```python
from build123d import *

# Parameters (mm, degrees)
F1_DEPTH      = 9
F2_R          = 5
F3_DEPTH      = 25
F4_W          = 103.9993347282
F4_H          = 56.6140824735
F5_DEPTH      = 25
F6_W          = 113.1558813547
F6_H          = 45.2373955332
F7_DEPTH      = 25
F8_R          = 5
F9_SIZE       = 5
F10_R         = 10
F11_T1_DEPTH  = 37.8584149398
F11_T3_DEPTH  = 109.8584149398
F11_T5_DEPTH  = 56.6140824735
F11_T7_DEPTH  = 104.1027474062
F11_T9_DEPTH  = 322.7168298797
F11_T11_DEPTH = 45.7168298797
F11_T13_DEPTH = 112.8584149398
F11_T15_DEPTH = 45.2373955332
F11_T17_DEPTH = 107.6210194067
F11_T19_DEPTH = 197
F11_T22_ANGLE = 90
F11_T24_ANGLE = 90
F11_T29_DEPTH = 122.7168298797
F11_T33_DEPTH = 69.4724974133
F11_T40_DEPTH = 69.4724974133
F11_T44_DEPTH = 122.7168298797
F11_T51_DEPTH = 58.095810473
F11_T55_DEPTH = 125.7168298797
F11_T62_DEPTH = 125.7168298797
F11_T66_DEPTH = 58.095810473


# Not quite as in the source:
# - a fillet or chamfer that OpenCascade refuses, or shapes differently, is made with other operations: its cross-section is extruded or revolved along the edge and cut away or added


with BuildPart() as f1:
    # F0 (on Front) → F1 (new body)
    with BuildSketch(Plane.XZ):
        with BuildLine():
            Line((100.0664040952, 56.5429037459), (-96.9335959048, 56.5429037459))
            ThreePointArc((-96.9335959048, 56.5429037459), (-132.2889349642, 41.8982428052), (-146.9335959048, 6.5429037459))
            Line((-146.9335959048, 6.5429037459), (-146.9335959048, -153.4570962541))
            Line((-146.9335959048, -153.4570962541), (150.0664040952, -153.4570962541))
            Line((150.0664040952, -153.4570962541), (150.0664040952, 6.5429037459))
            ThreePointArc((150.0664040952, 6.5429037459), (135.4217431545, 41.8982428052), (100.0664040952, 56.5429037459))
        make_face()
    extrude(amount=F1_DEPTH)

    # F2 (on face) → F3 (join)
    with BuildSketch(Plane.XZ.offset(9)):
        with Locations((-46.9335959048, -43.4570962541)):
            Circle(F2_R)
        with Locations((-96.9335959048, -43.4570962541)):
            Circle(F2_R)
    extrude(amount=F3_DEPTH)

    # F4 (on face) → F5 (cut)
    with BuildSketch(Plane.XZ.offset(9)):
        with Locations((105.0660714593, -46.7641374908)):
            Rectangle(F4_W, F4_H)
    extrude(amount=-F5_DEPTH, mode=Mode.SUBTRACT)

    # F6 (on face) → F7 (cut)
    with BuildSketch(Plane.XZ.offset(9)):
        with Locations((-103.5115365822, -110.8383984875)):
            Rectangle(F6_W, F6_H)
    extrude(amount=-F7_DEPTH, mode=Mode.SUBTRACT)

    # F8
    f8_edges = [f1.edges().sort_by_distance(p)[0] for p in [
        (150.066404, -9, -5.957096),
        (101.566404, -9, -18.457096),
        (53.066404, -9, -46.764137),
        (101.566404, -9, -75.071179),
        (150.066404, -9, -114.264137),
        (1.566404, -9, -153.457096),
        (-146.933596, -9, -143.457096),
        (-96.933596, -9, -133.457096),
        (-46.933596, -9, -110.838398),
        (-96.933596, -9, -88.219701),
        (-146.933596, -9, -40.838398),
        (-132.288935, -9, 41.898243),
        (1.566404, -9, 56.542904),
        (135.421743, -9, 41.898243),
        (-101.933596, -9, -43.457096),
        (-51.933596, -9, -43.457096),
    ]]
    fillet(f8_edges, radius=F8_R)

    # F9
    f9_edges = [f1.edges().sort_by_distance(p)[0] for p in [
        (-101.933596, -34, -43.457096),
        (-51.933596, -34, -43.457096),
    ]]
    chamfer(f9_edges, length=F9_SIZE)

    # F10
    f10_edges = [f1.edges().sort_by_distance(p)[0] for p in [
        (-94.433596, -31.5, -43.457096),
        (-101.933596, -29, -43.457096),
        (-44.433596, -31.5, -43.457096),
        (-51.933596, -29, -43.457096),
    ]]
    fillet(f10_edges, radius=F10_R)

    # F11: chamfer of 5 on 14 edges, made by hand

    # F11_s2 → F11_t1 (cut)
    with BuildSketch(Plane.XY.offset(-31.3155111939)):
        Polygon((150.0664040952, -5), (145.0664040952, 0), (150.0664040952, 0), align=None)
    extrude(amount=F11_T1_DEPTH, mode=Mode.SUBTRACT)

    # F11_s4 → F11_t3 (cut)
    with BuildSketch(Plane.YZ.offset(53.0664040952)):
        Polygon((-5, -18.4570962541), (0, -13.4570962541), (0, -18.4570962541), align=None)
        Polygon((-5, -75.0711787276), (0, -80.0711787276), (0, -75.0711787276), align=None)
    extrude(amount=F11_T3_DEPTH, mode=Mode.SUBTRACT)

    # F11_s6 → F11_t5 (cut)
    with BuildSketch(Plane.XY.offset(-75.0711787276)):
        Polygon((53.0664040952, -5), (48.0664040952, 0), (53.0664040952, 0), align=None)
    extrude(amount=F11_T5_DEPTH, mode=Mode.SUBTRACT)

    # F11_s8 → F11_t7 (cut)
    with BuildSketch(Plane.XY.offset(-166.3155111939)):
        Polygon((150.0664040952, -5), (145.0664040952, 0), (150.0664040952, 0), align=None)
    extrude(amount=F11_T7_DEPTH, mode=Mode.SUBTRACT)

    # F11_s10 → F11_t9 (cut)
    with BuildSketch(Plane.YZ.offset(-159.7920108447)):
        Polygon((-5, -153.4570962541), (0, -148.4570962541), (0, -153.4570962541), align=None)
    extrude(amount=F11_T9_DEPTH, mode=Mode.SUBTRACT)

    # F11_s12 → F11_t11 (cut)
    with BuildSketch(Plane.XY.offset(-166.3155111939)):
        Polygon((-146.9335959048, -5), (-141.9335959048, 0), (-146.9335959048, 0), align=None)
    extrude(amount=F11_T11_DEPTH, mode=Mode.SUBTRACT)

    # F11_s14 → F11_t13 (cut)
    with BuildSketch(Plane.YZ.offset(-159.7920108447)):
        Polygon((-5, -133.4570962541), (0, -138.4570962541), (0, -133.4570962541), align=None)
        Polygon((-5, -88.2197007209), (0, -83.2197007209), (0, -88.2197007209), align=None)
    extrude(amount=F11_T13_DEPTH, mode=Mode.SUBTRACT)

    # F11_s16 → F11_t15 (cut)
    with BuildSketch(Plane.XY.offset(-133.4570962541)):
        Polygon((-46.9335959048, -5), (-41.9335959048, 0), (-46.9335959048, 0), align=None)
    extrude(amount=F11_T15_DEPTH, mode=Mode.SUBTRACT)

    # F11_s18 → F11_t17 (cut)
    with BuildSketch(Plane.XY.offset(-101.0781156608)):
        Polygon((-146.9335959048, -5), (-141.9335959048, 0), (-146.9335959048, 0), align=None)
    extrude(amount=F11_T17_DEPTH, mode=Mode.SUBTRACT)

    # F11_s20 → F11_t19 (cut)
    with BuildSketch(Plane.YZ.offset(-96.9335959048)):
        Polygon((-5, 56.5429037459), (0, 51.5429037459), (0, 56.5429037459), align=None)
    extrude(amount=F11_T19_DEPTH, mode=Mode.SUBTRACT)

    # F11_s21 → F11_t22 (revolve, cut)
    with BuildSketch(Plane.YZ.offset(-96.9335959048)):
        Polygon((-5, 56.5429037459), (0, 51.5429037459), (0, 56.5429037459), align=None)
    revolve(axis=Axis((-96.9335959048, 0, 6.5429037459), (0, -1, 0)), revolution_arc=F11_T22_ANGLE, mode=Mode.SUBTRACT)

    # F11_s23 → F11_t24 (revolve, cut)
    with BuildSketch(Plane.XY.offset(6.5429037459)):
        Polygon((150.0664040952, -5), (145.0664040952, 0), (150.0664040952, 0), align=None)
    revolve(axis=Axis((100.0664040952, 0, 6.5429037459), (0, -1, 0)), revolution_arc=F11_T24_ANGLE, mode=Mode.SUBTRACT)


with BuildPart() as f11_tool27:
    # F11_s28 → F11_t29 (new body)
    with BuildSketch(Plane.YZ.offset(162.924819035)):
        Polygon((-5, -18.4570962541), (0, -13.4570962541), (0, -18.4570962541), align=None)
    extrude(amount=-F11_T29_DEPTH)

    split(bisect_by=Plane.YZ.offset(53.0664040952), keep=Keep.BOTTOM)


with BuildPart() as f11_tool31:
    # F11_s32 → F11_t33 (new body)
    with BuildSketch(Plane.XY.offset(-5.5986813143)):
        Polygon((53.0664040952, -5), (48.0664040952, 0), (53.0664040952, 0), align=None)
    extrude(amount=-F11_T33_DEPTH)

    split(bisect_by=Plane.XY.offset(-18.4570962541), keep=Keep.TOP)


with BuildPart() as f11_tool27_1:
    add(f11_tool27.part)

    # F11_t35: intersect F11_tool31
    add(f11_tool31.part, mode=Mode.INTERSECT)


with BuildPart() as f1_1:
    add(f1.part)

    # F11_t25: cut F11_tool27
    add(f11_tool27_1.part, mode=Mode.SUBTRACT)


with BuildPart() as f11_tool38:
    # F11_s39 → F11_t40 (new body)
    with BuildSketch(Plane.XY.offset(-18.4570962541)):
        Polygon((53.0664040952, -5), (48.0664040952, 0), (53.0664040952, 0), align=None)
    extrude(amount=-F11_T40_DEPTH)

    split(bisect_by=Plane.XY.offset(-75.0711787276), keep=Keep.BOTTOM)


with BuildPart() as f11_tool42:
    # F11_s43 → F11_t44 (new body)
    with BuildSketch(Plane.YZ.offset(40.2079891553)):
        Polygon((-5, -75.0711787276), (0, -80.0711787276), (0, -75.0711787276), align=None)
    extrude(amount=F11_T44_DEPTH)

    split(bisect_by=Plane.YZ.offset(53.0664040952), keep=Keep.BOTTOM)


with BuildPart() as f11_tool38_1:
    add(f11_tool38.part)

    # F11_t46: intersect F11_tool42
    add(f11_tool42.part, mode=Mode.INTERSECT)


with BuildPart() as f1_2:
    add(f1_1.part)

    # F11_t36: cut F11_tool38
    add(f11_tool38_1.part, mode=Mode.SUBTRACT)


with BuildPart() as f11_tool49:
    # F11_s50 → F11_t51 (new body)
    with BuildSketch(Plane.XY.offset(-146.3155111939)):
        Polygon((-46.9335959048, -5), (-41.9335959048, 0), (-46.9335959048, 0), align=None)
    extrude(amount=F11_T51_DEPTH)

    split(bisect_by=Plane.XY.offset(-133.4570962541), keep=Keep.BOTTOM)


with BuildPart() as f11_tool53:
    # F11_s54 → F11_t55 (new body)
    with BuildSketch(Plane.YZ.offset(-159.7920108447)):
        Polygon((-5, -133.4570962541), (0, -138.4570962541), (0, -133.4570962541), align=None)
    extrude(amount=F11_T55_DEPTH)

    split(bisect_by=Plane.YZ.offset(-46.9335959048), keep=Keep.TOP)


with BuildPart() as f11_tool49_1:
    add(f11_tool49.part)

    # F11_t57: intersect F11_tool53
    add(f11_tool53.part, mode=Mode.INTERSECT)


with BuildPart() as f1_3:
    add(f1_2.part)

    # F11_t47: cut F11_tool49
    add(f11_tool49_1.part, mode=Mode.SUBTRACT)


with BuildPart() as f11_tool60:
    # F11_s61 → F11_t62 (new body)
    with BuildSketch(Plane.YZ.offset(-34.075180965)):
        Polygon((-5, -88.2197007209), (0, -83.2197007209), (0, -88.2197007209), align=None)
    extrude(amount=-F11_T62_DEPTH)

    split(bisect_by=Plane.YZ.offset(-46.9335959048), keep=Keep.TOP)


with BuildPart() as f11_tool64:
    # F11_s65 → F11_t66 (new body)
    with BuildSketch(Plane.XY.offset(-133.4570962541)):
        Polygon((-46.9335959048, -5), (-41.9335959048, 0), (-46.9335959048, 0), align=None)
    extrude(amount=F11_T66_DEPTH)

    split(bisect_by=Plane.XY.offset(-88.2197007209), keep=Keep.TOP)


with BuildPart() as f11_tool60_1:
    add(f11_tool60.part)

    # F11_t68: intersect F11_tool64
    add(f11_tool64.part, mode=Mode.INTERSECT)


with BuildPart() as f1_4:
    add(f1_3.part)

    # F11_t58: cut F11_tool60
    add(f11_tool60_1.part, mode=Mode.SUBTRACT)


solid = f1_4.part
```
The model under review builds one solid part; all positions refer to its coordinate system, in mm. Round coordinates to 2 decimals unless told otherwise and drop trailing zeros. Order: outer loops, then holes, each group sorted by start corner. A loop starts at its lowest first (then second) coordinate and runs counter-clockwise, first axis right, second up. Notation, with made-up numbers: M -18.5,72 L -1.5,72 A26 cw -1.5,110 Z; hole C 17.25,26 d9. An arc over 180 degrees is marked long. Use a Markdown table: item, result.
1) Wall thickness on line 1 along Y through (x, z) = (-107.5, -29); line 2 along Z through (x, y) = (-97.5, -23); line 3 along Z through (x, y) = (61, -1.5): over which ranges is each line inside the solid? List them lowest first. Write a range as [from, to].
Report:
| item | result |
|---|---|
| line 1 | [-9, 0] |
| line 2 | [-48.42, -38.49] |
| line 3 | [-149.96, -78.57], [-14.96, 53.04] |
2) Consider section D-D (x = 36). Write out the cut boundary in (y, z).
Report:
| item | result |
|---|---|
| outline | M -9,-148.46 A5 ccw -4.92,-153.37 L 0,-148.46 L 0,51.54 L -4.92,56.46 A5 ccw -9,51.54 Z |
3) Consider section A-A (x = 95.5). Write out the cut boundary in (y, z).
Report:
| item | result |
|---|---|
| outline | M -9,-148.46 A5 ccw -4.92,-153.37 L 0,-148.46 L 0,-80.07 L -4.92,-75.16 A5 ccw -9,-80.07 Z; M -9,-13.46 A5 ccw -4.92,-18.37 L 0,-13.46 L 0,51.54 L -4.92,56.46 A5 ccw -9,51.54 Z |
4) Draft analysis for pull direction X (two halves, no side actions). For faces 1 (the face through (132.405, -0.239, 38.178)), 2 (the face through (-42.315, -19.353, -45.372)), 3 (the face through (0, 0, -47)), 4 (the face through (-101.93, -19.35, -43.24)), state which applies: released by +X, released by -X, zero draft, split by the parting line, or undercut.
Report:
| item | result |
|---|---|
| face 1 | released by +X |
| face 2 | undercut |
| face 3 | zero draft |
| face 4 | undercut |
5) Insertion check: pin 1 (2 mm diameter, centred on x = 33.5, y = -9.5, fed in from -Z); pin 2 (3 mm diameter, centred on x = 81.5, z = 9.5, fed in from -Y). Each pin has a flat end and moves straight along its axis. Give the tip position at first contact, or say it passes through.
Report:
| item | result |
|---|---|
| pin 1 | z = -150.64 |
| pin 2 | y = -9 |
6) Consider section C-C (y = -18). Write out the cut boundary in (x, z).
Report:
| item | result |
|---|---|
| outline | C -96.93,-43.46 d10; C -46.93,-43.46 d10 |
7) Consider section B-B (z = -111.5). Write out the cut boundary in (x, y).
Report:
| item | result |
|---|---|
| outline | M -46.85,-4.92 A5 ccw -41.93,-9 L 145.07,-9 A5 ccw 149.98,-4.92 L 145.07,0 L -41.93,0 Z |
